```python
from build123d import *

# Parameters (mm, degrees)
SKETCH_1_R      = 17.5
SKETCH_1_R_2    = 1.75
EXTRUDE_1_DEPTH = 3


with BuildPart() as part:
    # 草图1 → 凸台-拉伸1 (new body)
    with BuildSketch(Plane.XY):
        with BuildLine():
            ThreePointArc((-13.446268202, 20.480426545), (-20.859650045, 20.859650045), (-20.480426545, 13.446268202))
            ThreePointArc((-20.480426545, 13.446268202), (-24.5, 0), (-20.480426545, -13.446268202))
            ThreePointArc((-20.480426545, -13.446268202), (-20.859650045, -20.859650045), (-13.446268202, -20.480426545))
            ThreePointArc((-13.446268202, -20.480426545), (0, -24.5), (13.446268202, -20.480426545))
            ThreePointArc((13.446268202, -20.480426545), (20.859650045, -20.859650045), (20.480426545, -13.446268202))
            ThreePointArc((20.480426545, -13.446268202), (24.5, 0), (20.480426545, 13.446268202))
            ThreePointArc((20.480426545, 13.446268202), (20.859650045, 20.859650045), (13.446268202, 20.480426545))
            ThreePointArc((13.446268202, 20.480426545), (0, 24.5), (-13.446268202, 20.480426545))
        make_face()
        Circle(SKETCH_1_R, mode=Mode.SUBTRACT)
        with Locations((-17.324116139, 17.324116139)):
            Circle(SKETCH_1_R_2, mode=Mode.SUBTRACT)
        with Locations((17.324116139, 17.324116139)):
            Circle(SKETCH_1_R_2, mode=Mode.SUBTRACT)
        with Locations((17.324116139, -17.324116139)):
            Circle(SKETCH_1_R_2, mode=Mode.SUBTRACT)
        with Locations((-17.324116139, -17.324116139)):
            Circle(SKETCH_1_R_2, mode=Mode.SUBTRACT)
    extrude(amount=EXTRUDE_1_DEPTH)


solid = part.part
```
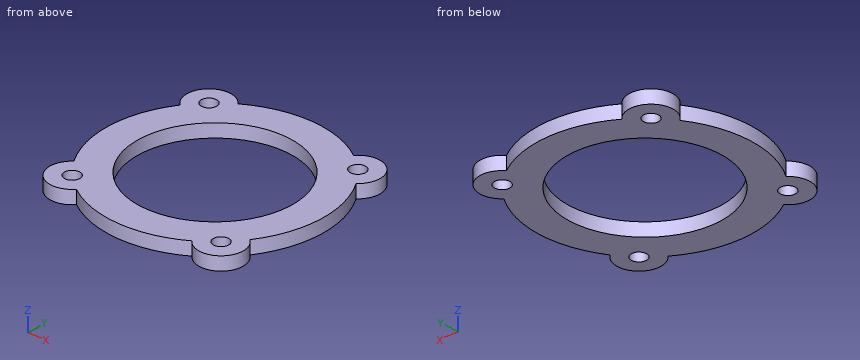
Geometry check sheet. Reference: the model listing, model coordinates, mm. Coordinates: 2 decimals unless noted, no trailing zeros. Loops run counter-clockwise (first coordinate to the right, second up) from the corner with the lowest first, then second, coordinate; pieces in that order, holes last. Notation, with made-up numbers: (-3.75, -11.75) -> (24.25, -11.75) arc R33 ccw to (24.25, 23.25) -> close; hole circle Ø7 at (63, 41). An arc over 180 degrees is marked (long way). Put each result on its own line as item: value.
1) Cross-section at C-C on z = 2.05. Record the boundary of the cut face in (x, y).
Result set:
outline: (-20.48, -13.45) arc R5 ccw (long way) to (-13.45, -20.48) arc R24.5 ccw to (13.45, -20.48) arc R5 ccw (long way) to (20.48, -13.45) arc R24.5 ccw to (20.48, 13.45) arc R5 ccw (long way) to (13.45, 20.48) arc R24.5 ccw to (-13.45, 20.48) arc R5 ccw (long way) to (-20.48, 13.45) arc R24.5 ccw to start; hole circle Ø3.5 at (-17.32, -17.32); hole circle Ø3.5 at (-17.32, 17.32); hole circle Ø35 at (0, 0); hole circle Ø3.5 at (17.32, -17.32); hole circle Ø3.5 at (17.32, 17.32)
2) Cross-section at A-A on x = 0. Record the boundary of the cut face in (y, z).
Result set:
outline: (-24.5, 0) -> (-17.5, 0) -> (-17.5, 3) -> (-24.5, 3) -> close; (17.5, 0) -> (24.5, 0) -> (24.5, 3) -> (17.5, 3) -> close
3) Thickness scan on line 1 (X direction, y = -18.5, z = 2.45); line 2 (Y direction, x = 0, z = 2.3); line 3 (X direction, y = 16, z = 1.6). Record the ranges inside material, lowest first.
Result set:
line 1: x = -22.18 to -18.62, -16.03 to 16.03, 18.62 to 22.18
line 2: y = -24.5 to -17.5, 17.5 to 24.5
line 3: x = -22.15 to -18.47, -16.18 to -7.09, 7.09 to 16.18, 18.47 to 22.15
4) Cross-section at B-B on y = -4.5. Record the boundary of the cut face in (x, z).
Result set:
outline: (-24.08, 0) -> (-16.91, 0) -> (-16.91, 3) -> (-24.08, 3) -> close; (16.91, 0) -> (24.08, 0) -> (24.08, 3) -> (16.91, 3) -> close
